Part print with two shaded views. Sizes in mm from the minimum x, y, z corner. A direction names the side the tool comes from. Coordinates: 2 decimals unless noted, no trailing zeros. Loops run counter-clockwise (first coordinate to the right, second up) from the corner with the lowest first, then second, coordinate; pieces in that order, holes last. Notation, with made-up numbers: (7.25, 8) -> (45.25, 8) arc R6 cw to (45.25, 18) -> close; hole circle Ø4 at (8.5, 23.25). An arc over 180 degrees is marked (long way). Write each question's results on one line, items separated by ' | '.
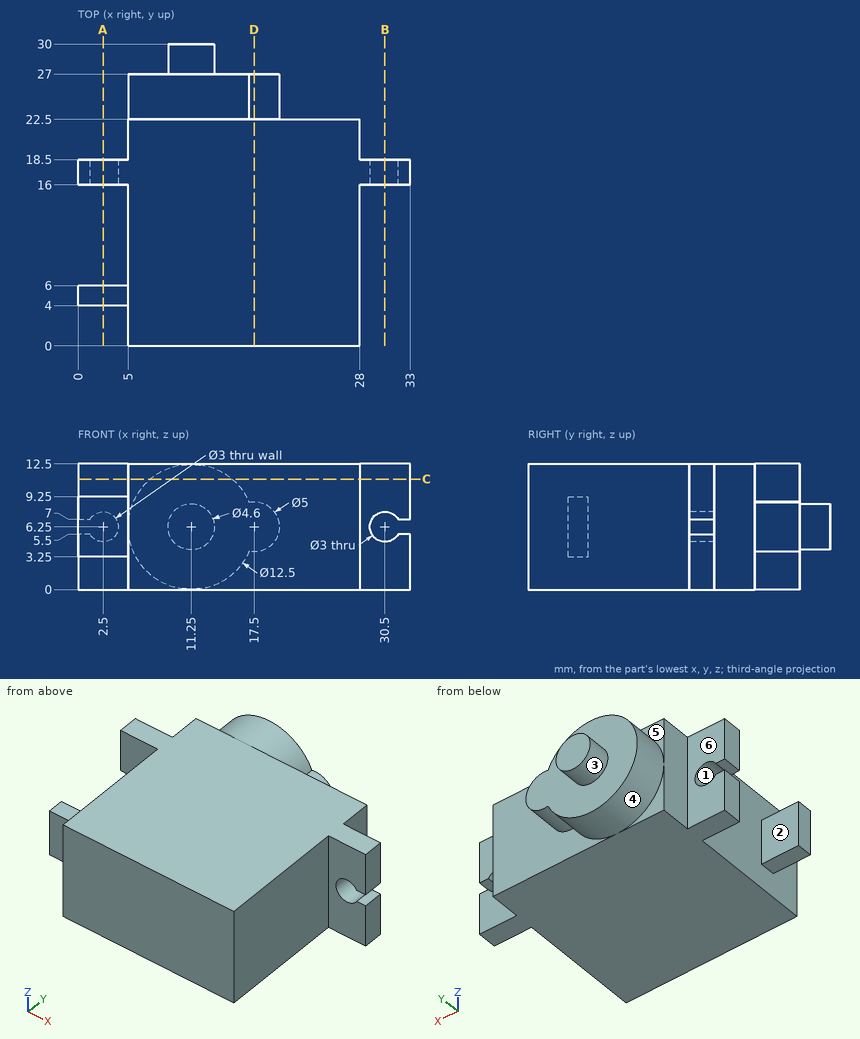
Q1. Cut at C-C on z = 11. Write the cut outline in (x, y).
Results are:
outline: (0, 16) -> (5, 16) -> (5, 0) -> (28, 0) -> (28, 16) -> (33, 16) -> (33, 18.5) -> (28, 18.5) -> (28, 22.5) -> (15.31, 22.5) -> (15.31, 27) -> (7.19, 27) -> (7.19, 22.5) -> (5, 22.5) -> (5, 18.5) -> (0, 18.5) -> close
Q2. Cut at D-D on x = 17.5. Write the cut outline in (y, z), and give its area (3 significant figures).
Results are:
outline: (0, 0) -> (22.5, 0) -> (22.5, 3.75) -> (27, 3.75) -> (27, 8.75) -> (22.5, 8.75) -> (22.5, 12.5) -> (0, 12.5) -> close | area: 304 mm^2
Q3. Cut at B-B on x = 30.5. Write the cut outline in (y, z).
Results are:
outline: (16, 0) -> (18.5, 0) -> (18.5, 4.75) -> (16, 4.75) -> close; (16, 7.75) -> (18.5, 7.75) -> (18.5, 12.5) -> (16, 12.5) -> close
Q4. Pull direction X, two halves, no side cores. Call the marked faces 1, 2 and 3: +X half, -X half, draft (parallel to the pull), parting line (faces both ways), or undercut.
Results are:
face 1: undercut | face 2: draft | face 3: parting line
Q5. Cut at A-A on x = 2.5. Write the cut outline in (y, z).
Results are:
outline: (4, 3.25) -> (6, 3.25) -> (6, 9.25) -> (4, 9.25) -> close; (16, 0) -> (18.5, 0) -> (18.5, 4.75) -> (16, 4.75) -> close; (16, 7.75) -> (18.5, 7.75) -> (18.5, 12.5) -> (16, 12.5) -> close
Q6. Wall check: L1, parallel to Z at x = 2.5, y = 17; L2, parallel to X at y = 16.6, z = 6.25; L3, parallel to Y at x = 9, z = 4.5. Give the ranges that are in metal, low to high. Write a range as from..to.
Results are:
L1: 0..4.75, 7.75..12.5 | L2: 4..29 | L3: 0..27
Q7. Drop flat-ended pins along their axis: pin 1 (1.5 mm diameter, centred on x = 2.5, z = 3.5, fed in from -Y); pin 2 (5 mm diameter, centred on x = 24, z = 5, fed in from -Y); pin 3 (1.5 mm diameter, centred on x = 2, z = 5, fed in from +Y); pin 4 (4 mm diameter, centred on x = 15.5, z = 3, fed in from +Y). Give the stop position or say it passes through.
Results are:
pin 1: y = 4 | pin 2: y = 0 | pin 3: y = 18.5 | pin 4: y = 27
Q8. Which spindle directions (+Z, -Z, +X, -X, +Y, -Y) get a long thin tool onto all of the face, cutting with end or side? Do the marked faces 4, 5 and 6. Say none if no direction does.
Results are:
face 4: +Y | face 5: +Z, -X, +Y | face 6: +Z, -Z, -X, +Y
